```python
from build123d import *

# Parameters (mm, degrees)
SKETCH_1_W               = 18
SKETCH_1_H               = 18
EXTRUDE_1_DEPTH          = 10
SKETCH_2_R               = 8.75
EXTRUDE_2_DEPTH          = 49.5
SKETCH_3_W               = 18
SKETCH_3_H               = 18
EXTRUDE_3_DEPTH          = 13
SKETCH_4_R               = 5
EXTRUDE_4_DEPTH          = 8
SKETCH_5_R               = 2.5
CUT_EXTRUDE_1_DEPTH      = 79.5
FILLET_1_R               = 5
CUT_EXTRUDE_2_REACH      = 84.977
CUT_EXTRUDE_2_END_RADIUS = 2.5
SKETCH_6_R               = 2.5


with BuildPart() as part:
    # 草图1 → 凸台-拉伸1 (new body)
    with BuildSketch(Plane.XY):
        Rectangle(SKETCH_1_W, SKETCH_1_H)
    extrude(amount=EXTRUDE_1_DEPTH)

    # 草图2 → 凸台-拉伸2 (add)
    with BuildSketch(Plane.XY.offset(10)):
        Circle(SKETCH_2_R)
    extrude(amount=EXTRUDE_2_DEPTH)

    # 草图3 → 凸台-拉伸3 (add)
    with BuildSketch(Plane.XY.offset(59.5)):
        Rectangle(SKETCH_3_W, SKETCH_3_H)
    extrude(amount=EXTRUDE_3_DEPTH)

    # 草图4 → 凸台-拉伸4 (add)
    with BuildSketch(Plane.XY.offset(72.5)):
        with Locations(Location((0, 0, 0), (0, 0, 180))):
            Circle(SKETCH_4_R)
    extrude(amount=EXTRUDE_4_DEPTH)

    # 草图5 → 切除-拉伸1 (cut)
    with BuildSketch(Plane.XY.offset(80.5)):
        Circle(SKETCH_5_R)
    extrude(amount=-CUT_EXTRUDE_1_DEPTH, mode=Mode.SUBTRACT)

    # 圆角1
    fillet_1_edges = [part.edges().sort_by_distance(p)[0] for p in [
        (9, -9, 66),
        (9, 9, 66),
        (-9, 9, 66),
        (-9, -9, 66),
        (9, -9, 5),
        (-9, -9, 5),
        (-9, 9, 5),
        (9, 9, 5),
    ]]
    fillet(fillet_1_edges, radius=FILLET_1_R)

    # 切除-拉伸2: up to this cylinder (the profile starts outside it)
    cut_extrude_2_end = Plane(origin=(0, 0, 34.75), z_dir=(0, 0, 1)) * Cylinder(CUT_EXTRUDE_2_END_RADIUS, 234.954, mode=Mode.PRIVATE)
    # 草图6 → 切除-拉伸2 (cut, up to the surface)
    with BuildSketch(Plane.XZ.offset(9), mode=Mode.PRIVATE) as cut_extrude_2_sk1:
        with Locations(Location((0, 5.25, 0), (0, 0, 270))):
            Circle(SKETCH_6_R)
    cut_extrude_2_tool1 = extrude(cut_extrude_2_sk1.sketch, amount=-CUT_EXTRUDE_2_REACH, mode=Mode.PRIVATE) - cut_extrude_2_end
    add(cut_extrude_2_tool1.solids().sort_by_distance((0, -9, 5.25))[0], mode=Mode.SUBTRACT)
    # 草图6 → 切除-拉伸2 (cut, up to the surface)
    with BuildSketch(Plane.XZ.offset(9), mode=Mode.PRIVATE) as cut_extrude_2_sk2:
        with Locations(Location((0, 64.25, 0), (0, 0, 270))):
            Circle(SKETCH_6_R)
    cut_extrude_2_tool2 = extrude(cut_extrude_2_sk2.sketch, amount=-CUT_EXTRUDE_2_REACH, mode=Mode.PRIVATE) - cut_extrude_2_end
    add(cut_extrude_2_tool2.solids().sort_by_distance((0, -9, 64.25))[0], mode=Mode.SUBTRACT)


solid = part.part
```
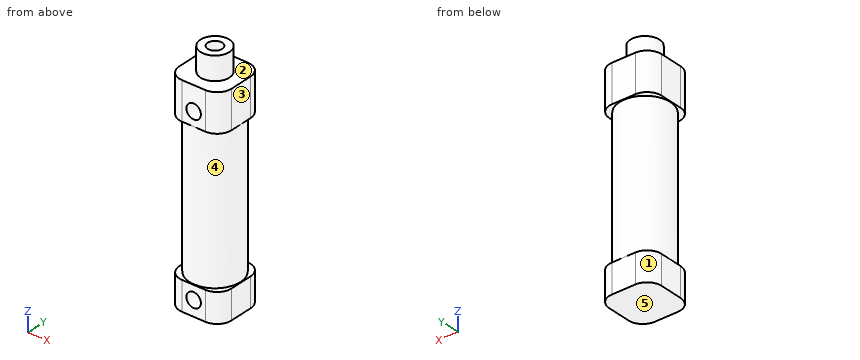
The model under review builds one solid part; all positions refer to its coordinate system, in mm. Face numbers are marked on the shaded views. A direction names the side the tool comes from. Round coordinates to 2 decimals unless told otherwise and drop trailing zeros. Write each loop counter-clockwise with the first axis right and the second up, starting at its lowest first coordinate (ties: lowest second). Pieces come first, ordered by that corner, then holes.
(1) We need section C-C on y = 6. Give the boundary of the cut face in (x, z), and give its area (3 significant figures).
(2) Mouldability with a two-part tool opening along Z and no side actions: class the marked faces 3, 4 and 5 as +Z half, -Z half, draft (parallel to the pull), parting line (faces both ways), or undercut.
(3) We need section B-B on z = 70. Give the boundary of the cut face in (x, y), and give its area (3 significant figures).
(4) We need section A-A on x = 0. Give the boundary of the cut face in (y, z).
(5) Insertion check: pin 1 (1.5 mm diameter, centred on x = -1.5, z = 15.5, fed in from +Y); pin 2 (5 mm diameter, centred on y = 5, z = 17.5, fed in from +X); pin 3 (3 mm diameter, centred on x = -5, z = 31, fed in from +Y). Each pin has a flat end and moves straight along its axis. Give the tip position at first contact, or say it passes through.
(6) Wall thickness on L1, parallel to X at y = -3.5, z = 5.25; L2, parallel to Y at x = -0.25, z = 29.5: over which ranges is each line inside the solid? List them lowest first.
(7) Machinability: for the marked faces 1 and 2, which of the approach directions +Z, -Z, +X, -X, +Y, -Y give a long, thin tool a straight path to every point of the face, cutting with its end or side? Answer none if there is none.
(8) We need section D-D on z = 14. Give the boundary of the cut face in (x, y).
Findings below:
1. outline: (-8.58, 0) - (8.58, 0) - (8.58, 10) - (6.37, 10) - (6.37, 59.5) - (8.58, 59.5) - (8.58, 72.5) - (-8.58, 72.5) - (-8.58, 59.5) - (-6.37, 59.5) - (-6.37, 10) - (-8.58, 10) - close
1. area: 1,030 mm2
2. face 3: draft
2. face 4: undercut
2. face 5: -Z half
3. outline: (-9, -4) arc R5 ccw to (-4, -9) - (4, -9) arc R5 ccw to (9, -4) - (9, 4) arc R5 ccw to (4, 9) - (-4, 9) arc R5 ccw to (-9, 4) - close; hole circle Ø5 at (0, 0)
3. area: 283 mm2
4. outline: (-9, 0) - (9, 0) - (9, 10) - (8.75, 10) - (8.75, 59.5) - (9, 59.5) - (9, 72.5) - (5, 72.5) - (5, 80.5) - (2.5, 80.5) - (2.5, 1) - (-2.5, 1) - (-2.5, 2.75) - (-9, 2.75) - close; (-9, 7.75) - (-2.5, 7.75) - (-2.5, 61.75) - (-9, 61.75) - (-9, 59.5) - (-8.75, 59.5) - (-8.75, 10) - (-9, 10) - close; (-9, 66.75) - (-2.5, 66.75) - (-2.5, 80.5) - (-5, 80.5) - (-5, 72.5) - (-9, 72.5) - close
5. pin 1: stops at y = 8.72
5. pin 2: stops at x = 8.39
5. pin 3: stops at y = 8.02
6. L1: x = -9 to -2.5, 2.5 to 9
6. L2: y = -8.75 to -2.49, 2.49 to 8.75
7. face 1: +Z, -Z, -X, +Y
7. face 2: +Z
8. outline: circle Ø17.5 at (0, 0); hole circle Ø5 at (0, 0)
